Autodesk Inventor part; units mm, degrees
ref_plane "YZ Plane" through (0, 0, 0) normal (1, 0, 0) x (0, 1, 0)
ref_plane "XZ Plane" through (0, 0, 0) normal (0, 1, 0) x (-1, 0, 0)
ref_plane "XY Plane" through (0, 0, 0) normal (0, 0, 1) x (1, 0, 0)
sketch "Sketch1" plane through (0, 0, 0) normal (0, 0, 1) x (1, 0, 0)
  circle A0 centre (0, 0) radius 6.35
  circle A1 centre (0, 0) radius 5.6388
  dimension "d0" = 12.7
  dimension "d1" = 11.2776
extrude "Extrusion1" add sketch "Sketch1" along normal blind 317.5
sketch "Sketch2" plane through (0, 0, 0) normal (0, 1, 0) x (-1, 0, 0)
  line L0 (0, 0) -> (0, 382.1904) construction
  circle A0 centre (0, 2.54) radius 1.6383
  circle A1 centre (0, 177.8) radius 1.6383
  line L1 (5.6388, 0) -> (-5.6388, 0)
  dimension "d4" = 3.2766
  dimension "d5" = 3.2766
  dimension "d6" = 2.54
  dimension "d10" = 177.8
extrude "Extrusion2" cut sketch "Sketch2" along normal through all both and the other way through all
equation "\"d4\" = d5"
properties part number "J001401" material "STAINLESS STEEL, 304"
Check sheet for the modelled part. Datum: model origin and axes. Units: mm. Round coordinates to 2 decimals unless told otherwise and drop trailing zeros. Order: outer loops, then holes, each group sorted by start corner. A loop starts at its lowest first (then second) coordinate and runs counter-clockwise, first axis right, second up. Notation, with made-up numbers: M 24.5,47.5 L 58.5,47.5 A13 ccw 58.5,56.5 Z; hole C -12.5,-31.5 d8. An arc over 180 degrees is marked long. One line per item, written item: value. Start each with the question number.
1. Section check B-B on z = 254. Enter the section's corners in (x, y).
2. Section check A-A on y = 0. Enter the section's corners in (x, z).
3. Scan lines: line 1 along Z through (x, y) = (0, -6.1); line 2 along Y through (x, z) = (0.5, 180); line 3 along Y through (x, z) = (2, 277). Record each from-to range of solid material in increasing order.
4. Gauge pin test, flat ends, axial feed: P1, Ø1, axis at x = -1, z = 196, coming from the +Y side; P2, Ø1, axis at y = 4.5, z = 138, coming from the -X side; P3, Ø4, axis at x = 3, z = 167.5, coming from the -Y side. Record the tip position at first contact, or that the pin passes through.
5. Release check for a two-part mould opening along Y. For faces 1 (the cylindrical face through (-1.38, 6.2, 156.53)), 2 (the flat face through (0, 6, 0)), 3 (the cylindrical face through (-1.222, 5.505, 156.528)) record: released by +Y, released by -Y, zero draft, split by the parting line, or undercut.
Results found:
1. outline: C 0,0 d12.7; hole C 0,0 d11.28
2. outline: M -6.35,0 L -5.64,0 L -5.64,317.5 L -6.35,317.5 Z; M 5.64,0 L 6.35,0 L 6.35,317.5 L 5.64,317.5 Z
3. line 1: 0 to 0.9, 4.18 to 176.16, 179.44 to 317.5
3. line 2: -6.33 to -5.62, 5.62 to 6.33
3. line 3: -6.03 to -5.27, 5.27 to 6.03
4. P1: y = 6.33
4. P2: x = -4.93
4. P3: y = -6.27
5. face 1: split by the parting line
5. face 2: zero draft
5. face 3: undercut
